The model under review builds one solid part; all positions refer to its coordinate system, in mm. Face numbers are marked on the shaded views. A direction names the side the tool comes from. Give positions to 0.01 mm unless a question says otherwise; leave off trailing zeros. Write each loop counter-clockwise with the first axis right and the second up, starting at its lowest first coordinate (ties: lowest second). Pieces come first, ordered by that corner, then holes. Notation, with made-up numbers: (24.25, 2) - (44.25, 2) arc R17 cw to (44.25, 31) - close; hole circle Ø7 at (-26, 5). An arc over 180 degrees is marked (long way). Write item = value, one per line.
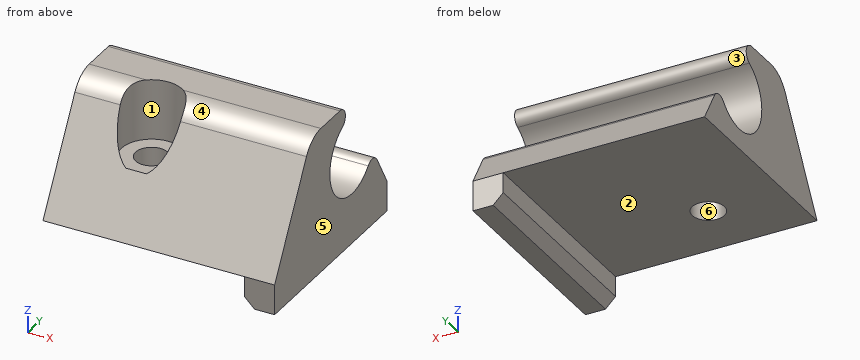
```python
from build123d import *

# Parameters (mm, degrees)
EXTRUDE_1_DEPTH      = 15.5
EXTRUDE_1_DEPTH_BACK = 7.5
SKETCH_2_R           = 1.6
CUT_EXTRUDE_1_DEPTH  = 25.050924737
SKETCH_3_R           = 3
CUT_EXTRUDE_2_DEPTH  = 6
SKETCH_4_W           = 3
SKETCH_4_H           = 20.350852961
EXTRUDE_2_DEPTH      = 3
FILLET_1_R           = 3
CHAMFER_2_SIZE       = 1


with BuildPart() as part:
    # 草图1 → 凸台-拉伸1 (new, two sides: drawn at the far end of the back side and taken through both)
    with BuildSketch(Plane(origin=(0, 0, 0), x_dir=(0, 0, -1), z_dir=(1, 0, 0)).offset(-EXTRUDE_1_DEPTH_BACK)):
        with BuildLine():
            Line((0, 0), (0, 14.350852961))
            Line((0, 14.350852961), (-3.11932209, 12.549911513))
            ThreePointArc((-3.11932209, 12.549911513), (-3.613338081, 11.79312076), (-3.295457672, 10.947108887))
            ThreePointArc((-3.295457672, 10.947108887), (-3.612312045, 4.790802869), (-9.6, 6.256440423))
            ThreePointArc((-9.6, 6.256440423), (-10.723606798, 6.795229963), (-11.5, 5.820550528))
            Line((-11.5, 5.820550528), (-11.5, 0.639528096))
            Line((-11.5, 0.639528096), (0, -6))
            Line((0, -6), (0, 0))
        make_face()
    extrude(amount=EXTRUDE_1_DEPTH + EXTRUDE_1_DEPTH_BACK)

    # 草图2 → 切除-拉伸1 (cut, through all)
    with BuildSketch(Plane.XY.offset(11.5)):
        Circle(SKETCH_2_R)
    extrude(amount=-CUT_EXTRUDE_1_DEPTH, mode=Mode.SUBTRACT)

    # 草图3 → 切除-拉伸2 (cut)
    with BuildSketch(Plane.XY.offset(11.5)):
        Circle(SKETCH_3_R)
    extrude(amount=-CUT_EXTRUDE_2_DEPTH, mode=Mode.SUBTRACT)

    # 草图4 → 凸台-拉伸2 (add)
    with BuildSketch(Plane(origin=(0, 0, 0), x_dir=(-1, 0, 0), z_dir=(0, 0, -1))):
        with Locations((-14, 4.175426481)):
            Rectangle(SKETCH_4_W, SKETCH_4_H)
    extrude(amount=EXTRUDE_2_DEPTH)

    # 圆角1
    fillet_1_edges = [part.edges().sort_by_distance(p)[0] for p in [
        (9.215520711, 0.639528096, 11.5),
        (-5.215520711, 0.639528096, 11.5),
    ]]
    fillet(fillet_1_edges, radius=FILLET_1_R)

    # 倒角2
    chamfer_2_edges = [part.edges().sort_by_distance(p)[0] for p in [
        (12.5, 4.175426481, -3),
    ]]
    chamfer(chamfer_2_edges, length=CHAMFER_2_SIZE)


solid = part.part
```
1. Take a section at C-C on z = -1.25. Give the boundary of the cut face in (x, y).
Findings below:
outline = (12.5, -6) - (15.5, -6) - (15.5, 14.35) - (12.5, 14.35) - close
2. Take a section at B-B on y = -3.75. Give the boundary of the cut face in (x, z), and give its area (3 significant figures).
Findings below:
outline = (-7.5, 0) - (12.5, 0) - (12.5, -2) - (13.5, -3) - (15.5, -3) - (15.5, 3.9) - (-7.5, 3.9) - close
area = 98.1 mm²
3. Machinability: for the marked faces 1, 2 and 3, which of the approach directions +Z, -Z, +X, -X, +Y, -Y give a long, thin tool a straight path to every point of the face, cutting with its end or side? Answer none if there is none.
Findings below:
face_1 = +Z
face_2 = -Z, -X, +Y, -Y
face_3 = +X, -X, +Y
4. Draft analysis for pull direction Y (two halves, no side actions). For the marked faces 4, 5 and 6, state which applies: +Y half, -Y half, draft (parallel to the pull), parting line (faces both ways), or undercut.
Findings below:
face_4 = -Y half
face_5 = draft
face_6 = undercut
5. For line 1 (X direction, y = 0, z = 10); line 2 (Z direction, x = 10.75, y = 8); line 3 (Z direction, x = -1.75, y = -1), list the stretches that pass through material, from the lowest coordinate up. Write a range as from..to.
Findings below:
line_1 = -7.5..-3, 3..15.5
line_2 = 0..2
line_3 = 0..5.5
6. Insertion check: P1, Ø3, axis at x = 1, y = -1, coming from the +Z side; P2, Ø1, axis at x = 11.5, z = 2, coming from the -Y side; P3, Ø5, axis at y = 8, z = 6, coming from the +X side; P4, Ø5, axis at x = 0, y = 0, coming from the -Z side. Each pin has a flat end and moves straight along its axis. Give the tip position at first contact, or say it passes through.
Findings below:
P1 = 5.5
P2 = -5.13
P3 = through
P4 = 0
7. Take a section at A-A on x = -0.5. Give the boundary of the cut face in (y, z).
Findings below:
outline = (-6, 0) - (-1.52, 0) - (-1.52, 5.5) - (-2.82, 5.5) - close; (1.52, 0) - (14.35, 0) - (12.55, 3.12) arc R1 ccw to (10.95, 3.3) arc R4 cw (long way) to (6.26, 9.6) arc R1 ccw to (5.82, 11.5) - (2.96, 11.5) - (2.96, 5.5) - (1.52, 5.5) - close
8. Take a section at D-D on x = 10.75. Give the boundary of the cut face in (y, z).
Findings below:
outline = (-6, 0) - (14.35, 0) - (12.55, 3.12) arc R1 ccw to (10.95, 3.3) arc R4 cw (long way) to (6.26, 9.6) arc R1 ccw to (5.82, 11.5) - (2.37, 11.5) arc R3 ccw to (-0.23, 10) - close
